Can you work these out from the model? Positions are in its coordinate system, mm. A direction names the side the tool comes from. Round coordinates to 2 decimals unless told otherwise and drop trailing zeros. Loops run counter-clockwise (first coordinate to the right, second up) from the corner with the lowest first, then second, coordinate; pieces in that order, holes last. Notation, with made-up numbers: M -18,48 L 5,48 A10 cw 5,52 Z; hole C -5,85 d1. An arc over 180 degrees is marked long. Answer as CSV lines item,"result".
from build123d import *

# Parameters (mm, degrees)
SCHIZZO1_W                    = 25
SCHIZZO1_H                    = 18
SCHIZZO1_W_2                  = 18
SCHIZZO1_W_3                  = 15
SCHIZZO1_H_2                  = 15
ESTRUSIONE_ESTRUSIONE1_DEPTH  = 15
TAGLIO_ESTRUSIONE1_DEPTH      = 42.291645644
TAGLIO_ESTRUSIONE1_DEPTH_BACK = 42.291645644
SCHIZZO2_R                    = 1.35
SCHIZZO3_R                    = 1.35
TAGLIO_ESTRUSIONE2_DEPTH      = 15
SCHIZZO4_R                    = 1.35
TAGLIO_ESTRUSIONE3_DEPTH      = 15


with BuildPart() as part:
    # Schizzo1 → Estrusione-Estrusione1 (new body)
    # profile 1 of 2: a face of its own
    with BuildSketch(Plane(origin=(0, 0, 0), x_dir=(0, 0, -1), z_dir=(1, 0, 0))):
        with Locations((-21.5, 0)):
            Rectangle(SCHIZZO1_W, SCHIZZO1_H)
    # profile 2 of 2: a face of its own
    with BuildSketch(Plane(origin=(0, 0, 0), x_dir=(0, 0, -1), z_dir=(1, 0, 0))):
        Rectangle(SCHIZZO1_W_2, SCHIZZO1_H)
        Rectangle(SCHIZZO1_W_3, SCHIZZO1_H_2, mode=Mode.SUBTRACT)
    extrude(amount=ESTRUSIONE_ESTRUSIONE1_DEPTH)

    # Schizzo2 → Taglio-Estrusione1 (cut, two sides: drawn at the far end of the back side and taken through both)
    with BuildSketch(Plane(origin=(0, 9, 0), x_dir=(1, 0, 0), z_dir=(0, 1, 0)).offset(-TAGLIO_ESTRUSIONE1_DEPTH_BACK)):
        with Locations(Location((7.5, -27, 0), (0, 0, 270))):
            Circle(SCHIZZO2_R)
        with Locations(Location((7.5, -23, 0), (0, 0, 270))):
            Circle(SCHIZZO2_R)
        with Locations(Location((7.5, -19, 0), (0, 0, 270))):
            Circle(SCHIZZO2_R)
        with Locations(Location((7.5, -15, 0), (0, 0, 270))):
            Circle(SCHIZZO2_R)
    extrude(amount=TAGLIO_ESTRUSIONE1_DEPTH + TAGLIO_ESTRUSIONE1_DEPTH_BACK, mode=Mode.SUBTRACT)

    # Schizzo3 → Taglio-Estrusione2 (cut)
    with BuildSketch(Plane(origin=(0, 9, 0), x_dir=(1, 0, 0), z_dir=(0, 1, 0))):
        with Locations(Location((7.5, -11, 0), (0, 0, 270))):
            Circle(SCHIZZO3_R)
    extrude(amount=-TAGLIO_ESTRUSIONE2_DEPTH, mode=Mode.SUBTRACT)

    # Schizzo4 → Taglio-Estrusione3 (cut)
    with BuildSketch(Plane.XZ.offset(9)):
        with Locations(Location((7.5, 31, 0), (0, 0, 270))):
            Circle(SCHIZZO4_R)
    extrude(amount=-TAGLIO_ESTRUSIONE3_DEPTH, mode=Mode.SUBTRACT)


solid = part.part
Item 1: We'd pull the mould along Y, two halves only. Please class faces 1 (the face through (8.839, 1.605, 10.824)), 2 (the face through (7, -7.5, 0)), 3 (the face through (7, -9, 13)): released by +Y, released by -Y, zero draft, split by the parting line, or undercut.
Output:
face 1,"zero draft"
face 2,"undercut"
face 3,"released by -Y"
Item 2: On a 3-axis mill with a long thin cutter (end or side, diameter ignored), from which of +Z, -Z, +X, -X, +Y, -Y can I reach the whole of each face in a straight line? I mean faces 4 (the face through (8, -6, 11)), 5 (the face through (7.906, -1.605, 29.712)), 6 (the face through (7, 0, 7.5)). Say none if no direction works.
Output:
face 4,"+Y"
face 5,"-Y"
face 6,"+X, -X"
Item 3: Will this pin go through, and if not, where does the flat tip stop? pin 1 (2.5 mm diameter, centred on x = 7.5, z = 19, fed in from -Y) (1 decimal).
Output:
pin 1,"passes through"
Item 4: If we section it at C-C on z = 27: Write out the boundary of the cut face in (x, y), then the cut area to 3 significant figures.
Output:
outline,"M 0,-9 L 6.15,-9 L 6.15,9 L 0,9 Z; M 8.85,-9 L 15,-9 L 15,9 L 8.85,9 Z"
area,"221 mm2"
Item 5: If I drill on line 1 along Y through (x, z) = (4, 2); line 2 along X through (y, z) = (4, 11); line 3 along Z through (x, y) = (10, -2), over which ranges is the centre line in solid material (lowest first)? Write a range as from..to.
Output:
line 1,"y = -9..-7.5, 7.5..9"
line 2,"x = 0..6.15, 8.85..15"
line 3,"z = -9..-7.5, 7.5..34"
Item 6: If we section it at B-B on x = 7.5: State how many separate pieces and enclosed holes the cut face has, then the cut area to 3 significant figures.
Output:
separate pieces,"5"
enclosed holes,"1"
area,"274 mm2"
Item 7: If we section it at D-D on x = 5.5: Write out the boundary of the cut face in (y, z), then the cut area to 3 significant figures.
Output:
outline,"M -9,-9 L 9,-9 L 9,34 L -9,34 Z; hole M -7.5,-7.5 L 7.5,-7.5 L 7.5,7.5 L -7.5,7.5 Z"
area,"549 mm2"
Item 8: If we section it at A-A on y = -3.5: Write out the boundary of the cut face in (x, z), then the cut area to 3 significant figures.
Output:
outline,"M 0,-9 L 15,-9 L 15,-7.5 L 0,-7.5 Z; M 0,7.5 L 15,7.5 L 15,34 L 0,34 Z; hole C 7.5,11 d2.7; hole C 7.5,15 d2.7; hole C 7.5,19 d2.7; hole C 7.5,23 d2.7; hole C 7.5,27 d2.7; hole C 7.5,31 d2.7"
area,"386 mm2"
